```python
from build123d import *

# Parameters (mm, degrees)
BOSS_EXTRUDE5_DEPTH = 67.31
CUT_EXTRUDE2_DEPTH  = 12.693340834
CUT_EXTRUDE3_DEPTH  = 25.4
CUT_EXTRUDE5_DEPTH  = 6.35
SKETCH16_W          = 6.35
SKETCH16_H          = 12.7
BOSS_EXTRUDE6_DEPTH = 12.7
SKETCH17_W          = 6.35
SKETCH17_H          = 12.7
CUT_EXTRUDE6_DEPTH  = 12.7
SKETCH18_R          = 2.8829
CUT_EXTRUDE7_DEPTH  = 12.7
SKETCH19_R          = 2.8829
CUT_EXTRUDE8_DEPTH  = 4.826
SKETCH21_R          = 2.8829
CUT_EXTRUDE9_DEPTH  = 4.826


with BuildPart() as part:
    # Sketch1 → Boss-Extrude5 (new body)
    with BuildSketch(Plane(origin=(0, 0, 0), x_dir=(1, 0, 0), z_dir=(0, 1, 0))):
        Polygon((-60.605605599, 37.663504972), (95.096394401, 37.663504972), (95.096394401, 18.613504972), (-41.555605599, 18.613504972), (-41.555605599, -118.038495028), (-60.605605599, -118.038495028), align=None)
    extrude(amount=BOSS_EXTRUDE5_DEPTH)

    # Sketch8 → Cut-Extrude2 (cut)
    with BuildSketch(Plane(origin=(0, 67.31, 0), x_dir=(1, 0, 0), z_dir=(0, 1, 0))):
        Polygon((-57.303605599, -118.038495028), (-57.303605599, 34.361504972), (95.096394401, 34.361504972), (95.096394401, 31.059504972), (-54.001605599, 31.059504972), (-54.001605599, -118.038495028), align=None)
    extrude(amount=-CUT_EXTRUDE2_DEPTH, mode=Mode.SUBTRACT)

    # Sketch9 → Cut-Extrude3 (cut)
    with BuildSketch(Plane(origin=(0, 67.31, 0), x_dir=(1, 0, 0), z_dir=(0, 1, 0))):
        Polygon((-49.683605599, -118.038495028), (-49.683605599, 26.741504972), (95.096394401, 26.741504972), (95.096394401, 18.613504972), (-41.555605599, 18.613504972), (-41.555605599, -118.038495028), align=None)
    extrude(amount=-CUT_EXTRUDE3_DEPTH, mode=Mode.SUBTRACT)

    # Sketch15 → Cut-Extrude5 (cut)
    with BuildSketch(Plane.XZ):
        Polygon((-41.555605599, 118.038495028), (-47.905605599, 118.038495028), (-47.905605599, -24.963504972), (95.096394401, -24.963504972), (95.096394401, -18.613504972), (-41.555605599, -18.613504972), align=None)
    extrude(amount=-CUT_EXTRUDE5_DEPTH, mode=Mode.SUBTRACT)

    # Sketch16 → Boss-Extrude6 (add)
    with BuildSketch(Plane.XY.offset(118.038495028)):
        with Locations((-44.730605599, 12.7)):
            Rectangle(SKETCH16_W, SKETCH16_H)
    extrude(amount=BOSS_EXTRUDE6_DEPTH)

    # Sketch17 → Cut-Extrude6 (cut)
    with BuildSketch(Plane(origin=(95.096394401, 0, 0), x_dir=(0, 0, -1), z_dir=(1, 0, 0))):
        with Locations((21.788504972, 12.7)):
            Rectangle(SKETCH17_W, SKETCH17_H)
    extrude(amount=-CUT_EXTRUDE6_DEPTH, mode=Mode.SUBTRACT)

    # Sketch18 → Cut-Extrude7 (cut)
    with BuildSketch(Plane(origin=(-41.555605599, 0, 0), x_dir=(0, 0, -1), z_dir=(1, 0, 0))):
        with Locations((-124.388495028, 12.7)):
            Circle(SKETCH18_R)
    extrude(amount=-CUT_EXTRUDE7_DEPTH, mode=Mode.SUBTRACT)

    # Sketch19 → Cut-Extrude8 (cut)
    with BuildSketch(Plane.XY.offset(-24.963504972)):
        with Locations((88.746394401, 12.7)):
            Circle(SKETCH19_R)
    extrude(amount=-CUT_EXTRUDE8_DEPTH, mode=Mode.SUBTRACT)

    # Sketch21 → Cut-Extrude9 (cut)
    with BuildSketch(Plane.XZ.offset(-6.35)):
        with Locations(Location((-44.730605599, -21.788504972, 0), (0, 0, 270))):
            Circle(SKETCH21_R)
    extrude(amount=-CUT_EXTRUDE9_DEPTH, mode=Mode.SUBTRACT)


solid = part.part
```
Work out the finished part from the listing and answer in its coordinate system (mm). A direction names the side the tool comes from. Give positions to 0.01 mm unless a question says otherwise; leave off trailing zeros. Order: outer loops, then holes, each group sorted by start corner. A loop starts at its lowest first (then second) coordinate and runs counter-clockwise, first axis right, second up.
1. Section D-D, the plane y = 35 is taken. Determine the outline of the cut face in (x, z).
Result sheet:
outline: (-60.61, -37.66) - (95.1, -37.66) - (95.1, -18.61) - (-41.56, -18.61) - (-41.56, 118.04) - (-60.61, 118.04) - close
2. For faces 1 (the flat face through (-41.556, 24, 55)), 2 (the flat face through (-46, 6.35, 18)), 3 (the cylindrical face through (-41.872, 8.729, -21.413)), 4 (the flat face through (22, 61, -31.06)), determine the directions among +Z, -Z, +X, -X, +Y, -Y from which every point of the face is accessible in a straight line to the end or side of a thin tool.
Result sheet:
face 1: +Z, +X, +Y, -Y
face 2: +Z, +X, -Y
face 3: -Y
face 4: +X, +Y
3. The mould has two halves that part along X. Classify faces 5 (the cylindrical face through (-44.686, 11.596, 121.725)), 6 (the flat face through (-57.304, 61, 43)), 7 (the flat face through (-49.684, 55, 47)), 8 (the flat face through (-15, 54.617, -32)): released by +X, released by -X, zero draft, split by the parting line, or undercut.
Result sheet:
face 5: zero draft
face 6: undercut
face 7: released by +X
face 8: undercut
4. Each of these flat-tipped pins is pushed along its axis until it touches: P1, Ø6.5, axis at x = -44.73, z = -21.79, coming from the -Y side; P2, Ø14, axis at x = -7, y = 58.5, coming from the +Z side; P3, Ø8, axis at x = -41, z = 0, coming from the -Y side; P4, Ø1.7, axis at x = 88.5, y = 14, coming from the +Z side. Where does it stop, or does it pass through?
Result sheet:
P1: stops at y = 0
P2: stops at z = -26.74
P3: stops at y = 6.35
P4: stops at z = -29.79
5. Straight lines are drawn through the part: L1, parallel to X at y = 60, z = -16; L2, parallel to Z at x = -40.5, y = 14; L3, parallel to X at y = 22, z = 47.5. For each, find the intervals that lie inside material, in ascending order.
Result sheet:
L1: x = -60.61 to -57.3, -54 to -49.68
L2: z = -37.66 to -18.61
L3: x = -60.61 to -41.56
6. Section A-A, the plane y = 60 is taken. Determine the outline of the cut face in (x, z), and give its area (3 significant figures).
Result sheet:
outline: (-60.61, -37.66) - (95.1, -37.66) - (95.1, -34.36) - (-57.3, -34.36) - (-57.3, 118.04) - (-60.61, 118.04) - close; (-54, -31.06) - (95.1, -31.06) - (95.1, -26.74) - (-49.68, -26.74) - (-49.68, 118.04) - (-54, 118.04) - close
area: 2,290 mm2
7. Section B-B, the plane z = 31.5 is taken. Determine the outline of the cut face in (x, y).
Result sheet:
outline: (-60.61, 0) - (-47.91, 0) - (-47.91, 6.35) - (-41.56, 6.35) - (-41.56, 41.91) - (-49.68, 41.91) - (-49.68, 67.31) - (-54, 67.31) - (-54, 54.62) - (-57.3, 54.62) - (-57.3, 67.31) - (-60.61, 67.31) - close
8. Section C-C, the plane x = -34 is taken. Determine the outline of the cut face in (y, z), and give its area (3 significant figures).
Result sheet:
outline: (0, -37.66) - (67.31, -37.66) - (67.31, -34.36) - (54.62, -34.36) - (54.62, -31.06) - (67.31, -31.06) - (67.31, -26.74) - (41.91, -26.74) - (41.91, -18.61) - (6.35, -18.61) - (6.35, -24.96) - (0, -24.96) - close
area: 994 mm2
